Autodesk Inventor part; units mm, degrees
ref_plane "YZ Plane" through (0, 0, 0) normal (1, 0, 0) x (0, 1, 0)
ref_plane "XZ Plane" through (0, 0, 0) normal (0, 1, 0) x (-1, 0, 0)
ref_plane "XY Plane" through (0, 0, 0) normal (0, 0, 1) x (1, 0, 0)
sketch "Sketch1" plane through (0, 0, 0) normal (0, 1, 0) x (-1, 0, 0)
  line L0 (0, 0) -> (-54.3, 0)
  line L1 (-54.3, 0) -> (-54.3, -65.9)
  line L2 (-54.3, -65.9) -> (0, -65.9)
  line L3 (0, -65.9) -> (0, 0)
  dimension "d0" = 54.3
  dimension "d1" = 65.9
extrude "Extrusion1" add sketch "Sketch1" along normal blind 1.6
sketch "Sketch2" plane through (0, 1.6, 0) normal (0, 1, 0) x (1, 0, 0)
  line L0 (0, 65.9) -> (0, 0)
  line L1 (54.3, 65.9) -> (0, 65.9)
  line L2 (54.3, 0) -> (54.3, 65.9)
  line L3 (0, 0) -> (54.3, 0)
  point P0 (4.2, 61.6)
  point P1 (50.3, 61.7)
  point P2 (4, 4.3)
  dimension "d4" = 4.2
  dimension "d5" = 4.3
  dimension "d6" = 4
  dimension "d7" = 4.2
  dimension "d8" = 4
  dimension "d9" = 4.3
hole "Hole1" at (4.2, 1.6, -61.6) at (50.3, 1.6, -61.7) at (4, 1.6, -4.3) direction (0, -1, 0) diameter 3.175 end through all
sketch "Sketch3" plane through (0, 1.6, 0) normal (0, 1, 0) x (1, 0, 0)
  line L0 (53.4872, 53.8448) -> (53.4872, 2.8448)
  line L1 (30.4872, 2.8448) -> (30.4872, 52.8828)
  line L2 (0, 0) -> (54.3, 0)
  line L3 (54.3, 0) -> (54.3, 65.9)
  line L4 (33.0272, 52.8828) -> (33.0272, 2.8448)
  line L5 (50.9472, 53.8448) -> (50.9472, 2.8448)
  line L6 (30.4872, 52.8828) -> (33.0272, 52.8828)
  line L7 (50.9472, 53.8448) -> (53.4872, 53.8448)
  line L8 (53.4872, 2.8448) -> (50.9472, 2.8448)
  line L9 (33.0272, 2.8448) -> (30.4872, 2.8448)
  dimension "d17" = 23
  dimension "d18" = 51
  dimension "d20" = 0.8128
  dimension "d21" = 2.54
  dimension "d22" = 2.54
extrude "Extrusion2" add sketch "Sketch3" along normal blind 5.08
sketch "Sketch4" plane through (0, 6.68, 0) normal (0, 1, 0) x (1, 0, 0)
  line L0 (30.4872, 52.8828) -> (30.4872, 2.8448)
  line L1 (30.4872, 2.8448) -> (33.0272, 2.8448)
  line L2 (33.0272, 2.8448) -> (33.0272, 52.8828)
  line L3 (33.0272, 52.8828) -> (30.4872, 52.8828)
  line L4 (53.4872, 2.8448) -> (53.4872, 53.8448)
  line L5 (50.9472, 53.8448) -> (50.9472, 2.8448)
  line L6 (50.9472, 2.8448) -> (53.4872, 2.8448)
  line L7 (53.4872, 53.8448) -> (50.9472, 53.8448)
  line L8 (30.4872, 52.8828) -> (30.4872, 2.8448)
  line L9 (30.4872, 52.8828) -> (53.4872, 52.8828)
  line L10 (53.4872, 52.8828) -> (53.4872, 2.8448)
  line L11 (53.4872, 2.8448) -> (30.4872, 2.8448)
  line L12 (30.4872, 2.8448) -> (30.4872, 52.8828)
  point P0 (0, 0)
extrude "Extrusion3" add sketch "Sketch4" along normal blind 1.6 contours L3 L2 L1 L0 | L9 L5 L11 L2 | L9 L4 L6 L5
sketch "Sketch5" plane through (0, 8.28, 0) normal (0, 1, 0) x (1, 0, 0)
  line L0 (45.4872, 47.7) -> (53.4872, 47.7)
  line L1 (53.4872, 47.7) -> (53.4872, 39.7)
  line L2 (53.4872, 39.7) -> (45.4872, 39.7)
  line L3 (45.4872, 39.7) -> (45.4872, 47.7)
  line L4 (53.4872, 2.8448) -> (53.4872, 52.8828)
  line L5 (53.4872, 52.8828) -> (30.4872, 52.8828)
  line L6 (0, 0) -> (54.3, 0)
  line L7 (30.4872, 52.8828) -> (30.4872, 2.8448)
  line L8 (30.4872, 2.8448) -> (53.4872, 2.8448)
  line L9 (53.4872, 2.8448) -> (53.4872, 52.8828)
  line L10 (53.4872, 52.8828) -> (30.4872, 52.8828)
  dimension "d27" = 8
  dimension "d28" = 8
  dimension "d61" = 39.7
extrude "Extrusion4" add sketch "Sketch5" along normal blind 6.4 contours L0 L1 L2 L3
sketch "Sketch7" plane through (0, 1.6, 0) normal (0, 1, 0) x (1, 0, 0)
  line L0 (1.016, 48.6) -> (6.096, 48.6)
  line L1 (6.096, 48.6) -> (6.096, 41)
  line L2 (6.096, 41) -> (1.016, 41)
  line L3 (1.016, 41) -> (1.016, 48.6)
  line L4 (54.3, 65.9) -> (0, 65.9)
  line L5 (0, 65.9) -> (0, 0)
  dimension "d32" = 5.08
  dimension "d33" = 7.6
  dimension "d34" = 17.3
  dimension "d35" = 1.016
extrude "Extrusion5" add sketch "Sketch7" along normal blind 2.5
sketch "Sketch8" plane through (0, 1.6, 0) normal (0, 1, 0) x (1, 0, 0)
  line L0 (11.4, 65.011) -> (17.268, 65.011)
  line L1 (17.268, 65.011) -> (17.268, 57.01)
  line L2 (17.268, 57.01) -> (11.4, 57.01)
  line L3 (11.4, 57.01) -> (11.4, 65.011)
  line L4 (0, 65.9) -> (0, 0)
  line L5 (54.3, 65.9) -> (0, 65.9)
  line L6 (20.5192, 65.011) -> (26.4, 65.011)
  line L7 (26.4, 65.011) -> (26.4, 57.01)
  line L8 (26.4, 57.01) -> (20.5192, 57.01)
  line L9 (20.5192, 57.01) -> (20.5192, 65.011)
  dimension "d39" = 8.001
  dimension "d40" = 11.4
  dimension "d41" = 0.889
  dimension "d43" = 8.001
  dimension "d44" = 3.2512
  dimension "d45" = 0.889
  dimension "d60" = 15
extrude "Extrusion6" add sketch "Sketch8" along normal blind 5.5
sketch "Sketch9" plane through (0, 1.6, 0) normal (0, 1, 0) x (1, 0, 0)
  line L0 (8.6868, 53.454) -> (28.6584, 53.454)
  line L1 (28.6584, 53.454) -> (28.6584, 0.6858)
  line L2 (28.6584, 0.6858) -> (8.6868, 0.6858)
  line L3 (8.6868, 0.6858) -> (8.6868, 53.454)
  line L4 (54.3, 65.9) -> (0, 65.9)
  line L5 (30.4872, 52.8828) -> (30.4872, 2.8448)
  line L6 (0, 65.9) -> (0, 0)
  line L7 (0, 0) -> (54.3, 0)
  dimension "d48" = 12.446
  dimension "d49" = 1.8288
  dimension "d50" = 8.6868
  dimension "d51" = 0.6858
extrude "Extrusion7" add sketch "Sketch9" along normal up to surface (6.68 mm away)
sketch "Sketch10" plane through (0, 0, 0) normal (0, -1, 0) x (1, 0, 0)
  line L0 (42.5398, -21.577) -> (24.1808, -21.577)
  line L1 (24.1808, -21.577) -> (24.1808, -12.2936)
  line L2 (24.1808, -12.2936) -> (42.5398, -12.2936)
  line L3 (42.5398, -12.2936) -> (42.5398, -21.577)
  line L4 (54.3, -65.9) -> (0, -65.9)
  line L5 (54.3, 0) -> (54.3, -65.9)
  line L6 (0, -65.9) -> (0, 0)
  line L7 (0, 0) -> (54.3, 0)
  dimension "d54" = 44.323
  dimension "d55" = 11.7602
  dimension "d56" = 24.1808
  dimension "d57" = 12.2936
extrude "Extrusion8" add sketch "Sketch10" along normal blind 1.016 contours L0 L1 L2 L3
properties part number "PCB"
Read the model definition and answer for the solid it produces. Units are mm, in the model's axes. A direction names the side the tool comes from. Coordinates: 2 decimals unless noted, no trailing zeros. Order: outer loops, then holes, each group sorted by start corner. A loop starts at its lowest first (then second) coordinate and runs counter-clockwise, first axis right, second up. Notation, with made-up numbers: M 60.25,5.25 L 114.25,5.25 A9 ccw 114.25,22.25 Z; hole C 10.25,73.25 d5. An arc over 180 degrees is marked long. Put each result on its own line as item: value. Start each with the question number.
Item 1: Section B-B, the plane z = -45 is taken. Determine the outline of the cut face in (x, y), plus the area to 3 significant figures.
Item 2: For faces 1 (the face through (34, 1.6, -40)), 2 (the face through (11.4, 4, -61)), 3 (the face through (30.487, 5, -28)), 4 (the face through (4, 4.1, -45)), 5 (the face through (42, 6.68, -28)), determine the directions among +Z, -Z, +X, -X, +Y, -Y from which every point of the face is accessible in a straight line to the end or side of a thin tool.
Item 3: Given pin 1 Ø1.2 at (y, z) = (3, -46.5) entering from +X; pin 2 Ø2.5 at (x, z) = (4, -4.3) entering from -Y; pin 3 Ø1.6 at (x, y) = (24.5, 4) entering from -Z; pin 4 Ø2 at (x, y) = (3.5, 3) entering from -Z, each flat-ended and moving along its own axis, determine where each tip first touches the part or whether it passes through.
Item 4: Section C-C, the plane z = -15.5 is taken. Determine the outline of the cut face in (x, y), plus the area to 3 significant figures.
Item 5: Consider probe 1 along Z at (x, y) = (4.2, 1.15); probe 2 along X at (y, z) = (0.8, -61.7); probe 3 along Y at (x, z) = (42, -22). Determine where each line is inside the solid, lowest interval first. Write a range as [from, to].
Item 6: The mould has two halves that part along Z. Classify faces 6 (the face through (28, 1, -65.9)), 7 (the face through (23, 7.1, -61)), 8 (the face through (14, 4, -57.01)): +Z half, -Z half, draft (parallel to the pull), parting line (faces both ways), or undercut.
Item 7: Section D-D, the plane z = -61.7 is taken. Determine the outline of the cut face in (x, y), plus the area to 3 significant figures.
Item 8: Section A-A, the plane z = -4.3 is taken. Determine the outline of the cut face in (x, y).
Computed:
1. outline: M 0,0 L 54.3,0 L 54.3,1.6 L 53.49,1.6 L 53.49,14.68 L 45.49,14.68 L 45.49,8.28 L 30.49,8.28 L 30.49,1.6 L 28.66,1.6 L 28.66,8.28 L 8.69,8.28 L 8.69,1.6 L 6.1,1.6 L 6.1,4.1 L 1.02,4.1 L 1.02,1.6 L 0,1.6 Z; hole M 33.03,1.6 L 50.95,1.6 L 50.95,6.68 L 33.03,6.68 Z
1. area: 347 mm2
2. face 1: none
2. face 2: -Z, -X, +Y
2. face 3: +Z, -Z, +Y
2. face 4: +Z, -Z, -X, +Y
2. face 5: +Z, -Z
3. pin 1: stops at x = 53.49
3. pin 2: passes through
3. pin 3: stops at z = -65.01
3. pin 4: stops at z = -48.6
4. outline: M 0,0 L 24.18,0 L 24.18,-1.02 L 42.54,-1.02 L 42.54,0 L 54.3,0 L 54.3,1.6 L 53.49,1.6 L 53.49,8.28 L 30.49,8.28 L 30.49,1.6 L 28.66,1.6 L 28.66,8.28 L 8.69,8.28 L 8.69,1.6 L 0,1.6 Z; hole M 33.03,1.6 L 50.95,1.6 L 50.95,6.68 L 33.03,6.68 Z
4. area: 302 mm2
5. probe 1: z = [-65.9, -63.19], [-60.01, -5.87], [-2.73, 0]
5. probe 2: x = [0, 2.62], [5.78, 48.71], [51.89, 54.3]
5. probe 3: y = [0, 1.6], [6.68, 8.28]
6. face 6: -Z half
6. face 7: draft
6. face 8: undercut
7. outline: M 0,0 L 2.62,0 L 2.62,1.6 L 0,1.6 Z; M 5.78,0 L 48.71,0 L 48.71,1.6 L 26.4,1.6 L 26.4,7.1 L 20.52,7.1 L 20.52,1.6 L 17.27,1.6 L 17.27,7.1 L 11.4,7.1 L 11.4,1.6 L 5.78,1.6 Z; M 51.89,0 L 54.3,0 L 54.3,1.6 L 51.89,1.6 Z
7. area: 141 mm2
8. outline: M 0,0 L 2.41,0 L 2.41,1.6 L 0,1.6 Z; M 5.59,0 L 54.3,0 L 54.3,1.6 L 53.49,1.6 L 53.49,8.28 L 30.49,8.28 L 30.49,1.6 L 28.66,1.6 L 28.66,8.28 L 8.69,8.28 L 8.69,1.6 L 5.59,1.6 Z; hole M 33.03,1.6 L 50.95,1.6 L 50.95,6.68 L 33.03,6.68 Z
